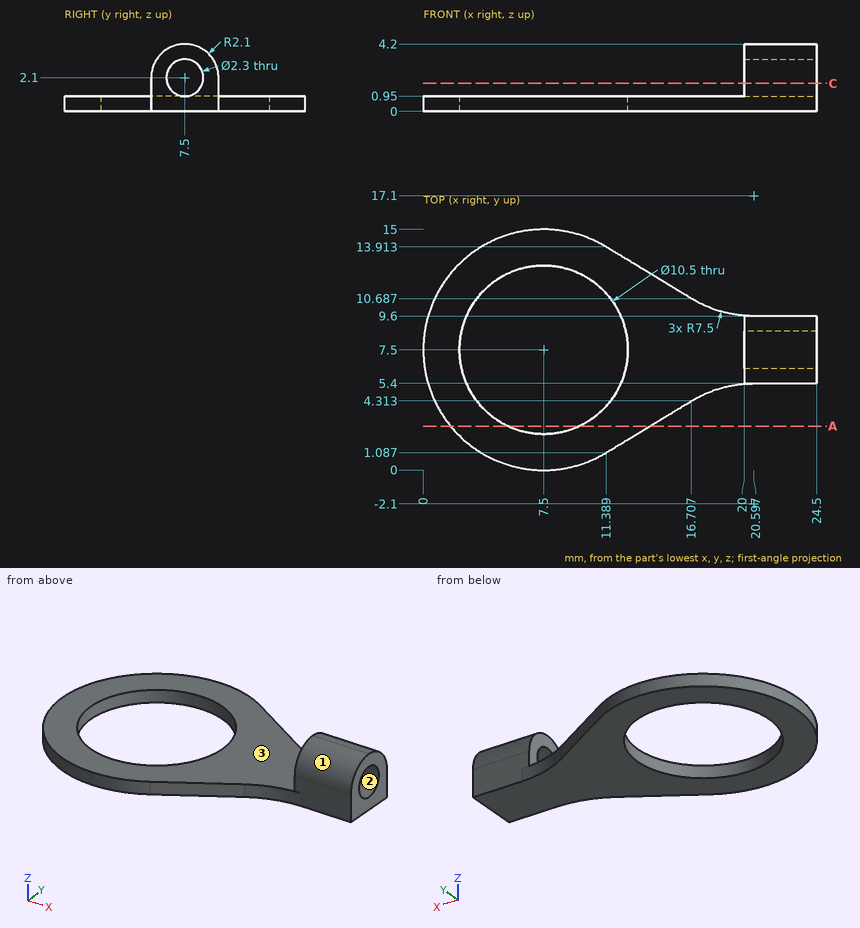
Here's the drawing with two shaded views (mm, measured from the low corner). I have some questions. Coordinates: 2 decimals unless noted, no trailing zeros. Order: outer loops, then holes, each group sorted by start corner. A loop starts at its lowest first (then second) coordinate and runs counter-clockwise, first axis right, second up. Notation, with made-up numbers: (50, 8) - (78, 8) arc R17 ccw to (78, 30) - close; hole circle Ø8 at (-37.5, 82). An arc over 180 degrees is marked (long way). Answer in a Markdown table with one row per item.
1. Suppose I cut it at C-C (z = 1.75). Please give me the cut outline in (x, y) (1 decimal).
Reply:
| item | result |
|---|---|
| outline | (20, 5.4) - (24.5, 5.4) - (24.5, 6.4) - (20, 6.4) - close; (20, 8.6) - (24.5, 8.6) - (24.5, 9.6) - (20, 9.6) - close |
2. Suppose I cut it at A-A (y = 2.75). Please give me the cut outline in (x, z).
Reply:
| item | result |
|---|---|
| outline | (1.7, 0) - (5.26, 0) - (5.26, 0.95) - (1.7, 0.95) - close; (9.74, 0) - (14.13, 0) - (14.13, 0.95) - (9.74, 0.95) - close |
3. For pin 1 (6 mm diameter, centred on x = 16, y = 2.5, fed in from +Z); pin 2 (1.4 mm diameter, centred on y = 7.5, z = 2.1, fed in from -X); pin 3 (2.5 mm diameter, centred on y = 8, z = 2.5, fed in from -X); pin 4 (1.7 mm diameter, centred on x = 23, z = 1, fed in from -Y), each with a flat end and sliding along its axis, tell me the tip position at first contact or that it passes through.
Reply:
| item | result |
|---|---|
| pin 1 | stops at z = 0.95 |
| pin 2 | passes through |
| pin 3 | stops at x = 20 |
| pin 4 | stops at y = 5.4 |
4. If we mould it in two halves opening along Y, with no side actions, what happens to the marked faces 1, 2 and 3? For each: pulls with the +Y half, pulls with the -Y half, needs draft (parallel to the pull), parting line crosses it, or undercut.
Reply:
| item | result |
|---|---|
| face 1 | pulls with the -Y half |
| face 2 | undercut |
| face 3 | needs draft |
5. If I drill on line 1 along X through (y, z) = (7.5, 0.4); line 2 along Z through (x, y) = (21.9, 7.5); line 3 along Y through (x, z) = (21.55, 2.1), over which ranges is the centre line in solid material (lowest first)?
Reply:
| item | result |
|---|---|
| line 1 | x = 0 to 2.25, 12.75 to 24.5 |
| line 2 | z = 0 to 0.95, 3.25 to 4.2 |
| line 3 | y = 5.4 to 6.35, 8.65 to 9.6 |
